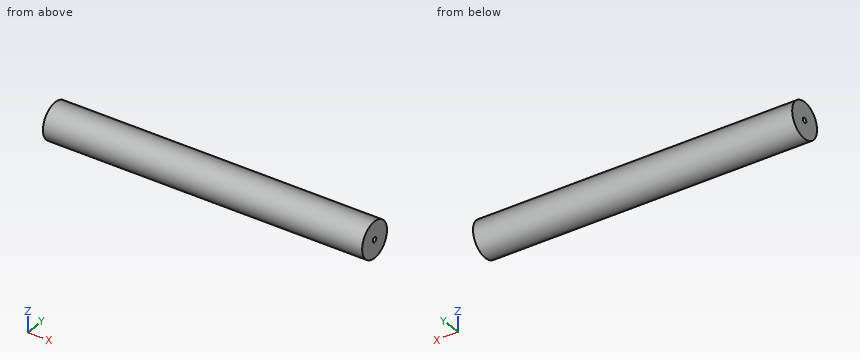
Autodesk Inventor part; units mm, degrees
ref_plane "YZ Plane" through (0, 0, 0) normal (1, 0, 0) x (0, 1, 0)
ref_plane "XZ Plane" through (0, 0, 0) normal (0, 1, 0) x (-1, 0, 0)
ref_plane "XY Plane" through (0, 0, 0) normal (0, 0, 1) x (1, 0, 0)
sketch "Sketch1" plane through (0, 0, 0) normal (0, 0, 1) x (1, 0, 0)
  point P0 (0, 0)
sketch "Sketch2" plane through (0, 0, 0) normal (1, 0, 0) x (0, 1, 0)
  circle A0 centre (0, 0) radius 14.2875
  dimension "d0" = 28.575
extrude "Extrusion1" add sketch "Sketch2" along normal mid plane 254
sketch "Sketch3" plane through (127, 0, 0) normal (1, 0, 0) x (0, 0, -1)
  point P0 (0, 0)
  point P1 (0, 0)
sketch "Sketch4" plane through (-127, 0, 0) normal (-1, 0, 0) x (0, 0, 1)
  point P0 (0, 0)
  point P1 (0, 0)
hole "Hole1" at (127, 0, 0) direction (-1, 0, 0) diameter 3.9624 depth 13.6144 tip angle 118
hole "Hole2" at (-127, 0, 0) direction (1, 0, 0) diameter 3.9624 depth 13.6144 tip angle 118
properties part number "CL2-002" material "Aluminum 6061"
For this review, take the finished solid that the model builds, in its own axes (mm). Give positions to 0.01 mm unless a question says otherwise; leave off trailing zeros. Order: outer loops, then holes, each group sorted by start corner. A loop starts at its lowest first (then second) coordinate and runs counter-clockwise, first axis right, second up.
1) Take a section at C-C (z = 10.5). Give the boundary of the cut face in (x, y).
2) Wall thickness on line 1 (Z direction, x = 124.25, y = 0); line 2 (Y direction, x = -96, z = 1); line 3 (Z direction, x = 49.5, y = -2.25): over which ranges is each line inside the solid? List them lowest first.
3) Take a section at B-B (y = -5). Give the boundary of the cut face in (x, z).
4) Take a section at A-A (x = -36). Give the boundary of the cut face in (y, z) (1 decimal), then the cut area to 3 significant figures.
5) Insertion check: pin 1 (4 mm diameter, centred on x = 6, z = -10.5, fed in from -Y); pin 2 (3 mm diameter, centred on x = -57.5, z = -3, fed in from -Y); pin 3 (3 mm diameter, centred on x = -20, z = -9, fed in from +Y); pin 4 (10 mm diameter, centred on y = 0, z = -1, fed in from +X). Each pin has a flat end and moves straight along its axis. Give the tip position at first contact, or say it passes through.
Derived:
1. outline: (-127, -9.69) - (127, -9.69) - (127, 9.69) - (-127, 9.69) - close
2. line 1: z = -14.29 to -1.98, 1.98 to 14.29
2. line 2: y = -14.25 to 14.25
2. line 3: z = -14.11 to 14.11
3. outline: (-127, -13.38) - (127, -13.38) - (127, 13.38) - (-127, 13.38) - close
4. outline: circle Ø28.6 at (0, 0)
4. area: 641 mm2
5. pin 1: stops at y = -11.48
5. pin 2: stops at y = -14.21
5. pin 3: stops at y = 12.16
5. pin 4: stops at x = 127
